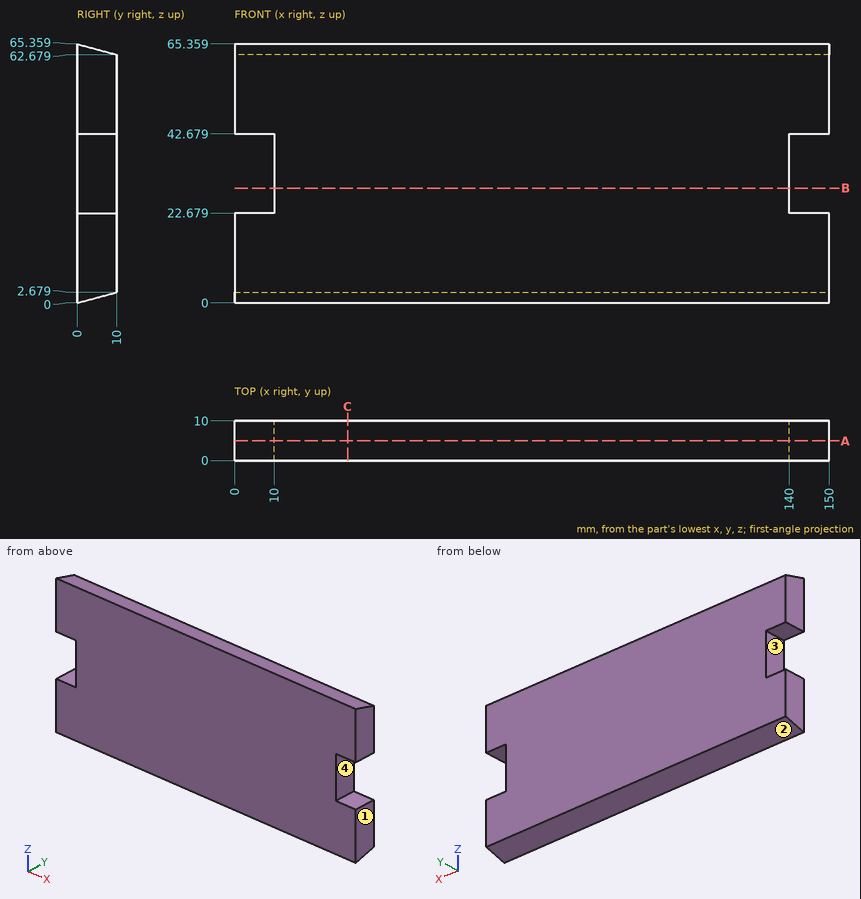
Can you work these out from the drawing? Everything is in mm from the part's minimum corner. Round coordinates to 2 decimals unless told otherwise and drop trailing zeros. Write each loop counter-clockwise with the first axis right and the second up, starting at its lowest first coordinate (ties: lowest second). Pieces come first, ordered by that corner, then holes. Notation, with made-up numbers: (-11.75, -37) - (-0.75, -37) arc R22 cw to (-0.75, -20) - close; hole circle Ø8 at (28.5, 85). An arc over 180 degrees is marked (long way). Put each result on its own line as item: value. Start each with the question number.
(1) Will these pins go through, and if not, where does the flat tip stop? pin 1 (3 mm diameter, centred on x = 143.5, y = 4, fed in from +Z); pin 2 (3 mm diameter, centred on y = 7, z = 37, fed in from +X); pin 3 (5 mm diameter, centred on x = 143.5, y = 3, fed in from -Z).
(2) I want a section at A-A, the plane y = 5. Please give me the cut outline in (x, z), plus the area to 3 significant figures.
(3) Thinking about a two-plate mould opening in Z: for the marked faces 1, 2, 3 and 4, which applies, released by +Z, released by -Z, zero draft, split by the parting line, or undercut?
(4) I want a section at B-B, the plane z = 29. Please give me the cut outline in (x, y).
(5) I need wall thicknesses on probe 1 along X at (y, z) = (6.75, 26); probe 2 along Z at (x, y) = (144.5, 1.5); probe 3 along Z at (x, y) = (75, 2) (1 decimal). Which ranges of each line are inside material? Lowest first, please.
(6) I want a section at C-C, the plane x = 28.5. Please give me the cut outline in (y, z), plus the area to 3 significant figures.
Here are the results:
1. pin 1: stops at z = 64.69
1. pin 2: stops at x = 140
1. pin 3: stops at z = 0.13
2. outline: (0, 1.34) - (150, 1.34) - (150, 22.68) - (140, 22.68) - (140, 42.68) - (150, 42.68) - (150, 64.02) - (0, 64.02) - (0, 42.68) - (10, 42.68) - (10, 22.68) - (0, 22.68) - close
2. area: 9,000 mm^2
3. face 1: zero draft
3. face 2: released by -Z
3. face 3: undercut
3. face 4: undercut
4. outline: (10, 0) - (140, 0) - (140, 10) - (10, 10) - close
5. probe 1: x = 10 to 140
5. probe 2: z = 0.4 to 22.68, 42.68 to 64.96
5. probe 3: z = 0.5 to 64.8
6. outline: (0, 0) - (10, 2.68) - (10, 62.68) - (0, 65.36) - close
6. area: 627 mm^2
